Read the model definition and answer for the solid it produces. Units are mm, in the model's axes. A direction names the side the tool comes from. Give positions to 0.01 mm unless a question says otherwise; leave off trailing zeros. Write each loop counter-clockwise with the first axis right and the second up, starting at its lowest first coordinate (ties: lowest second). Pieces come first, ordered by that corner, then holes. Notation, with made-up numbers: (32.25, -35.75) -> (73.25, -35.75) arc R20 cw to (73.25, -31.75) -> close; hole circle Ø6 at (62, 26). An arc over 180 degrees is marked (long way). Use a Markdown table: item, result.
from build123d import *

# Parameters (mm, degrees)
SKETCH1_W           = 300
SKETCH1_H           = 300
BOSS_EXTRUDE1_DEPTH = 260
FILLET1_R           = 20
SKETCH2_W           = 250
SKETCH2_H           = 250
CUT_EXTRUDE1_DEPTH  = 240
SKETCH3_R           = 5.5
CUT_EXTRUDE2_DEPTH  = 25
SKETCH4_W           = 5
SKETCH4_H           = 5
CUT_EXTRUDE3_DEPTH  = 25
SKETCH6_W           = 5
SKETCH6_H           = 5
CUT_EXTRUDE4_DEPTH  = 25
SKETCH7_W           = 5
SKETCH7_H           = 5
CUT_EXTRUDE5_DEPTH  = 25
SKETCH8_W           = 5
SKETCH8_H           = 5
CUT_EXTRUDE6_DEPTH  = 25
SKETCH9_W           = 5
SKETCH9_H           = 5
CUT_EXTRUDE7_DEPTH  = 20


with BuildPart() as part:
    # Sketch1 → Boss-Extrude1 (new body)
    with BuildSketch(Plane.XY):
        with Locations((150, 150)):
            Rectangle(SKETCH1_W, SKETCH1_H)
    extrude(amount=BOSS_EXTRUDE1_DEPTH)

    # Fillet1
    fillet1_edges = [part.edges().sort_by_distance(p)[0] for p in [
        (150, 300, 0),
        (300, 150, 0),
        (150, 0, 0),
        (0, 150, 0),
        (0, 300, 130),
        (300, 300, 130),
        (300, 0, 130),
        (0, 0, 130),
    ]]
    fillet(fillet1_edges, radius=FILLET1_R)

    # Sketch2 → Cut-Extrude1 (cut)
    with BuildSketch(Plane.XY.offset(260)):
        with Locations((150, 150)):
            Rectangle(SKETCH2_W, SKETCH2_H)
    extrude(amount=-CUT_EXTRUDE1_DEPTH, mode=Mode.SUBTRACT)

    # Sketch3 → Cut-Extrude2 (cut)
    with BuildSketch(Plane(origin=(0, 300, 0), x_dir=(1, 0, 0), z_dir=(0, 1, 0))):
        with Locations(Location((150, -150, 0), (0, 0, 270))):
            Circle(SKETCH3_R)
    extrude(amount=-CUT_EXTRUDE2_DEPTH, mode=Mode.SUBTRACT)

    # Sketch4 → Cut-Extrude3 (cut)
    with BuildSketch(Plane(origin=(0, 300, 0), x_dir=(1, 0, 0), z_dir=(0, 1, 0))):
        with Locations((70, -70)):
            Rectangle(SKETCH4_W, SKETCH4_H)
        with Locations((70, -210)):
            Rectangle(SKETCH4_W, SKETCH4_H)
        with Locations((230, -70)):
            Rectangle(SKETCH4_W, SKETCH4_H)
        with Locations((230, -210)):
            Rectangle(SKETCH4_W, SKETCH4_H)
    extrude(amount=-CUT_EXTRUDE3_DEPTH, mode=Mode.SUBTRACT)

    # Sketch6 → Cut-Extrude4 (cut)
    with BuildSketch(Plane(origin=(300, 0, 0), x_dir=(0, 0, -1), z_dir=(1, 0, 0))):
        with Locations((-210, 230)):
            Rectangle(SKETCH6_W, SKETCH6_H)
        with Locations((-210, 70)):
            Rectangle(SKETCH6_W, SKETCH6_H)
        with Locations((-70, 230)):
            Rectangle(SKETCH6_W, SKETCH6_H)
        with Locations((-70, 70)):
            Rectangle(SKETCH6_W, SKETCH6_H)
    extrude(amount=-CUT_EXTRUDE4_DEPTH, mode=Mode.SUBTRACT)

    # Sketch7 → Cut-Extrude5 (cut)
    with BuildSketch(Plane.XZ):
        with Locations((70, 210)):
            Rectangle(SKETCH7_W, SKETCH7_H)
        with Locations((70, 70)):
            Rectangle(SKETCH7_W, SKETCH7_H)
        with Locations((230, 210)):
            Rectangle(SKETCH7_W, SKETCH7_H)
        with Locations((230, 70)):
            Rectangle(SKETCH7_W, SKETCH7_H)
    extrude(amount=-CUT_EXTRUDE5_DEPTH, mode=Mode.SUBTRACT)

    # Sketch8 → Cut-Extrude6 (cut)
    with BuildSketch(Plane.ZY):
        with Locations((70, 230)):
            Rectangle(SKETCH8_W, SKETCH8_H)
        with Locations((70, 70)):
            Rectangle(SKETCH8_W, SKETCH8_H)
        with Locations((210, 230)):
            Rectangle(SKETCH8_W, SKETCH8_H)
        with Locations((210, 70)):
            Rectangle(SKETCH8_W, SKETCH8_H)
    extrude(amount=-CUT_EXTRUDE6_DEPTH, mode=Mode.SUBTRACT)

    # Sketch9 → Cut-Extrude7 (cut)
    with BuildSketch(Plane(origin=(0, 0, 0), x_dir=(-1, 0, 0), z_dir=(0, 0, -1))):
        with Locations((-230, 230)):
            Rectangle(SKETCH9_W, SKETCH9_H)
        with Locations((-230, 70)):
            Rectangle(SKETCH9_W, SKETCH9_H)
        with Locations((-70, 230)):
            Rectangle(SKETCH9_W, SKETCH9_H)
        with Locations((-70, 70)):
            Rectangle(SKETCH9_W, SKETCH9_H)
    extrude(amount=-CUT_EXTRUDE7_DEPTH, mode=Mode.SUBTRACT)


solid = part.part
Item 1: A cutting plane is placed at A-A (x = 150). Give the vertices of the cut face in (y, z).
Return value:
| item | result |
|---|---|
| outline | (0, 20) arc R20 ccw to (20, 0) -> (280, 0) arc R20 ccw to (300, 20) -> (300, 144.5) -> (275, 144.5) -> (275, 20) -> (25, 20) -> (25, 260) -> (0, 260) -> close; (275, 155.5) -> (300, 155.5) -> (300, 260) -> (275, 260) -> close |
Item 2: A tool of negligible diameter and unlimited length cuts with its end or side. For faces 1 (the face through (148, 275, 142)), 2 (the face through (148, 300, 138)), 3 (the face through (150.242, 287.675, 144.505)), from which of +Z, -Z, +X, -X, +Y, -Y can it reach the whole face along a straight path? Write none if from no direction.
Return value:
| item | result |
|---|---|
| face 1 | +Z |
| face 2 | +Z, -Z, +X, -X, +Y |
| face 3 | +Y |
Item 3: A cutting plane is placed at B-B (z = 42). Give the vertices of the cut face in (x, y), then the cut area to 3 significant figures.
Return value:
| item | result |
|---|---|
| outline | (0, 20) arc R20 ccw to (20, 0) -> (280, 0) arc R20 ccw to (300, 20) -> (300, 280) arc R20 ccw to (280, 300) -> (20, 300) arc R20 ccw to (0, 280) -> close; hole (25, 25) -> (275, 25) -> (275, 275) -> (25, 275) -> close |
| area | 27,200 mm^2 |
Item 4: A cutting plane is placed at D-D (z = 150). Give the vertices of the cut face in (x, y), then the cut area to 3 significant figures.
Return value:
| item | result |
|---|---|
| outline | (0, 20) arc R20 ccw to (20, 0) -> (280, 0) arc R20 ccw to (300, 20) -> (300, 280) arc R20 ccw to (280, 300) -> (155.5, 300) -> (155.5, 275) -> (275, 275) -> (275, 25) -> (25, 25) -> (25, 275) -> (144.5, 275) -> (144.5, 300) -> (20, 300) arc R20 ccw to (0, 280) -> close |
| area | 26,900 mm^2 |
Item 5: A cutting plane is placed at C-C (x = 221). Give the vertices of the cut face in (y, z).
Return value:
| item | result |
|---|---|
| outline | (0, 20) arc R20 ccw to (20, 0) -> (280, 0) arc R20 ccw to (300, 20) -> (300, 260) -> (275, 260) -> (275, 20) -> (25, 20) -> (25, 260) -> (0, 260) -> close |
Item 6: Straight lines are drawn through the part: line 1 along X through (y, z) = (266, 123); line 2 along X through (y, z) = (287.5, 150). For each, find the intervals that lie inside material, in ascending order. Write a range as [from, to].
Return value:
| item | result |
|---|---|
| line 1 | [0, 25], [275, 300] |
| line 2 | [1.46, 144.5], [155.5, 298.54] |
Item 7: For a pull along Y with two mould halves and no side action, classify faces 4 (the face through (294.297, 293.986, 141.68)), 5 (the face through (0, 148, 138)), 6 (the face through (275, 148, 142)) as +Y half, -Y half, draft (parallel to the pull), parting line (faces both ways), or undercut.
Return value:
| item | result |
|---|---|
| face 4 | +Y half |
| face 5 | draft |
| face 6 | undercut |
Item 8: Each of these flat-tipped pins is pushed along its axis until it touches: P1, Ø5.5, axis at y = 285, z = 70.5, coming from the +X side; P2, Ø2.5, axis at y = 15, z = 70, coming from the +X side; P3, Ø4, axis at y = 287, z = 69.5, coming from the +X side. Where does it stop, or does it pass through?
Return value:
| item | result |
|---|---|
| P1 | x = 299.87 |
| P2 | x = 299.65 |
| P3 | x = 299.36 |
